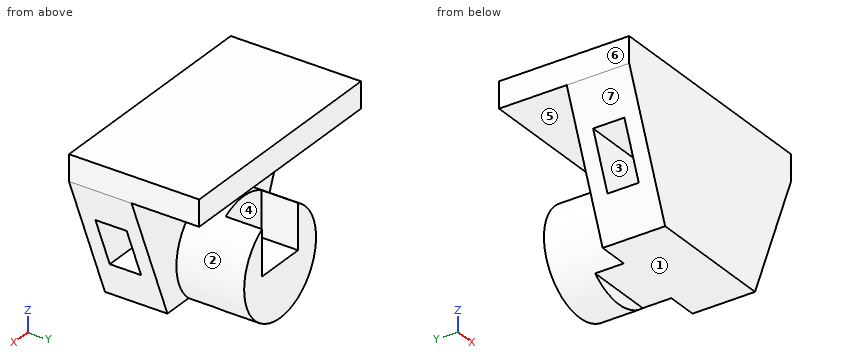
Autodesk Inventor part; units mm, degrees
ref_plane "YZ Plane" through (0, 0, 0) normal (1, 0, 0) x (0, 1, 0)
ref_plane "XZ Plane" through (0, 0, 0) normal (0, 1, 0) x (-1, 0, 0)
ref_plane "XY Plane" through (0, 0, 0) normal (0, 0, 1) x (1, 0, 0)
sketch "Szkic1" plane through (0, 0, 0) normal (0, 0, 1) x (1, 0, 0)
  line L0 (0, 0) -> (90, 0)
  line L1 (90, 0) -> (90, 50)
  line L2 (90, 50) -> (0, 50)
  line L3 (0, 50) -> (0, 0)
  dimension "d0" = 90
  dimension "d1" = 50
extrude "Wyciągnięcie proste1" add sketch "Szkic1" along normal blind 10
sketch "Szkic2" plane through (0, 0, 0) normal (0, -1, 0) x (1, 0, 0)
  line L0 (90, 0) -> (0, 0)
  line L1 (20, -50) -> (70, -50)
  line L2 (70, -50) -> (90, 0)
  line L3 (90, 0) -> (0, 0)
  line L4 (0, 0) -> (0, 10)
  line L5 (20, -50) -> (0, 0)
  line L6 (0, 0) -> (90, 0)
  dimension "d6" = 50
extrude "Wyciągnięcie proste2" add sketch "Szkic2" against normal blind 24
sketch "Szkic3" plane through (0, 24, 0) normal (0, 1, 0) x (1, 0, 0)
  line L0 (0, 0) -> (0, -10)
  line L1 (90, 0) -> (0, 0)
  circle A0 centre (45, 35) radius 20
  dimension "d11" = 40
extrude "Wyciągnięcie proste3" add sketch "Szkic3" along normal blind 26
sketch "Szkic4" plane through (0, 0, 10) normal (0, -1, 0) x (1, 0, 0)
  line L0 (70, -60) -> (58.2288, -60)
  line L1 (70, -60) -> (70, -66.9782)
  line L2 (70, -66.9782) -> (20, -66.9782)
  line L3 (31.7712, -60) -> (20, -60)
  line L4 (20, -66.9782) -> (20, -60)
  line L5 (20, -60) -> (70, -60)
  point P0 (0, -10)
extrude "Wyciągnięcie proste4" cut sketch "Szkic4" against normal blind 35
sketch "Szkic5" plane through (0, 0, 10) normal (-1, 0, 0) x (0, 0, 1)
  line L0 (-25, 6) -> (-25, 18)
  line L1 (-25, 18) -> (-45, 18)
  line L2 (-45, 18) -> (-45, 6)
  line L3 (-45, 6) -> (-25, 6)
  point P0 (-10, 0)
  dimension "d18" = 12
  dimension "d19" = 20
extrude "Wyciągnięcie proste5" cut sketch "Szkic5" against normal blind 95
sketch "Szkic6" plane through (45, 50, -35) normal (0, 1, 0) x (1, 0, 0)
  line L0 (-31, 0) -> (31, 0)
  line L1 (0, 0) -> (10, 0)
  line L2 (10, 0) -> (10, -28.0711)
  line L3 (10, -28.0711) -> (-10, -28.0711)
  line L4 (-10, -28.0711) -> (-10, 0)
  line L5 (-10, 0) -> (0, 0)
  point P0 (-45, -35)
  dimension "d22" = 10
  dimension "d23" = 20
extrude "Wyciągnięcie proste6" cut sketch "Szkic6" against normal blind 14
Build history of the part. All positions in model axes, mm. Face numbers are marked on the shaded views. A direction names the side the tool comes from. Round coordinates to 2 decimals unless told otherwise and drop trailing zeros. Write each loop counter-clockwise with the first axis right and the second up, starting at its lowest first coordinate (ties: lowest second). Pieces come first, ordered by that corner, then holes. Notation, with made-up numbers: M 4.5,-6.5 L 25.5,-6.5 A10 cw 25.5,11.5 Z; hole C 58,-10 d7. An arc over 180 degrees is marked long. Answer in a Markdown table with one row per item.
1. Mould opens along Z. For the marked faces 4, 5, 6 and 7 say: +Z half, -Z half, draft (parallel to the pull), parting line (faces both ways), or undercut.
Geometry check:
| item | result |
|---|---|
| face 4 | undercut |
| face 5 | undercut |
| face 6 | draft |
| face 7 | -Z half |
2. Probe L1, parallel to Y at x = 61, z = -29.5; L2, parallel to Z at x = 55, y = 31; L3, parallel to Y at x = 25.5, z = -4. List the from-to ranges inside material, lowest first. Write a range as [from, to].
Geometry check:
| item | result |
|---|---|
| L1 | [0, 6], [18, 50] |
| L2 | [-50, -17.68], [0, 10] |
| L3 | [0, 24] |
3. Saw through at C-C (z = -21). List the corners of the cut face in (x, y), and give its area (3 significant figures).
Geometry check:
| item | result |
|---|---|
| outline | M 8.4,0 L 81.6,0 L 81.6,6 L 8.4,6 Z; M 8.4,18 L 81.6,18 L 81.6,24 L 59.28,24 L 59.28,50 L 55,50 L 55,36 L 35,36 L 35,50 L 30.72,50 L 30.72,24 L 8.4,24 Z |
| area | 1,340 mm2 |
4. Saw through at D-D (x = 9). List the corners of the cut face in (y, z), and give its area (3 significant figures).
Geometry check:
| item | result |
|---|---|
| outline | M 0,-22.5 L 6,-22.5 L 6,-15 L 18,-15 L 18,-22.5 L 24,-22.5 L 24,0 L 50,0 L 50,10 L 0,10 Z |
| area | 950 mm2 |
5. Flat gauge pins, fed straight in: P1, Ø1.5, axis at x = 49.5, z = -52, coming from the -Y side; P2, Ø12, axis at y = 34.5, z = -16, coming from the -X side; P3, Ø2, axis at y = 15, z = -13, coming from the -X side. Where does each tip first touch, or does it go through?
Geometry check:
| item | result |
|---|---|
| P1 | y = 35 |
| P2 | x = 29.8 |
| P3 | x = 4.8 |
6. Saw through at B-B (x = 67.5). List the corners of the cut face in (y, z), and give its area (3 significant figures).
Geometry check:
| item | result |
|---|---|
| outline | M 0,-50 L 24,-50 L 24,0 L 50,0 L 50,10 L 0,10 Z; hole M 6,-35 L 18,-35 L 18,-15 L 6,-15 Z |
| area | 1,460 mm2 |
7. Saw through at A-A (y = 38). List the corners of the cut face in (x, z), and give its area (3 significant figures).
Geometry check:
| item | result |
|---|---|
| outline | M 0,0 L 90,0 L 90,10 L 0,10 Z; M 35,-35 L 35,-17.68 A20 ccw long 55,-17.68 L 55,-35 Z |
| area | 1,770 mm2 |
8. Which spindle directions (+Z, -Z, +X, -X, +Y, -Y) get a long thin tool onto all of the face, cutting with end or side? Do the marked faces 1, 2 and 3. Say none if no direction does.
Geometry check:
| item | result |
|---|---|
| face 1 | -Z, +X, -X, -Y |
| face 2 | +Y |
| face 3 | +X, -X |
